Check sheet for the drawn part. Datum: minimum x, y, z corner. Units: mm. A direction names the side the tool comes from. Round coordinates to 2 decimals unless told otherwise and drop trailing zeros. Order: outer loops, then holes, each group sorted by start corner. A loop starts at its lowest first (then second) coordinate and runs counter-clockwise, first axis right, second up. Notation, with made-up numbers: M 1,-1.75 L 43,-1.75 A11 cw 43,11.25 Z; hole C 84.25,34.25 d10. An arc over 180 degrees is marked long. Answer as a JSON object with one key per item and string values. Group by question number.
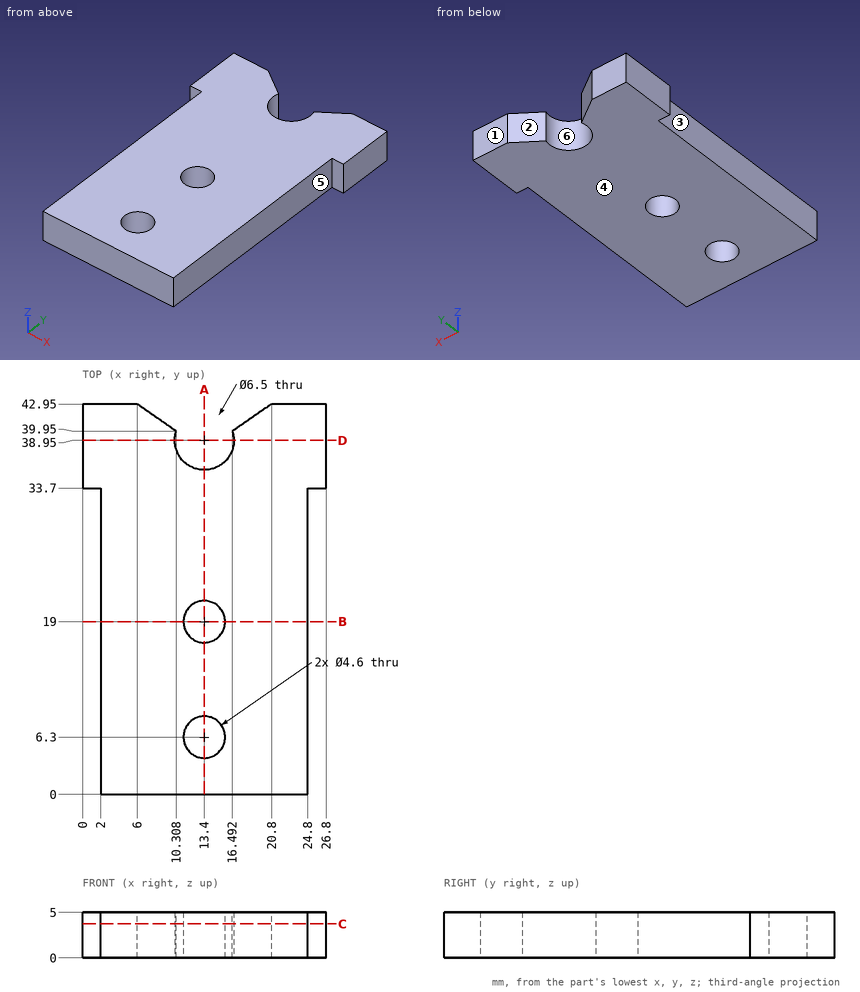
1) Go/stop test with flat-tipped pins: P1, Ø1, axis at x = 18.5, z = 3.5, coming from the +Y side; P2, Ø1.6, axis at x = 26, z = 2, coming from the -Y side; P3, Ø1.5, axis at y = 11, z = 3, coming from the -X side. Record where each tip stops, or that it passes through.
2) Set-up check for the marked faces 1, 2 and 3: record each of +Z, -Z, +X, -X, +Y, -Y from which the full face is reachable in a straight line by a thin tool's end or side.
3) Sectioned sample at A-A (x = 13.4). Record the boundary of the cut face in (y, z).
4) Release check for a two-part mould opening along X. For the marked faces 4, 5 and 6 record: +X half, -X half, draft (parallel to the pull), parting line (faces both ways), or undercut.
5) Thickness scan on line 1 along Y through (x, z) = (13.4, 2.9); line 2 along X through (y, z) = (6.5, 3.3); line 3 along Y through (x, z) = (15.5, 1.1) (1 decimal). Record the ranges inside material, lowest first. Write a range as [from, to].
6) Sectioned sample at D-D (y = 38.95). Record the boundary of the cut face in (x, z), then the cut area to 4 significant figures.
7) Sectioned sample at C-C (z = 3.75). Record the boundary of the cut face in (x, y).
8) Sectioned sample at B-B (y = 19). Record the boundary of the cut face in (x, z), then the cut area to 3 significant figures.
Final values:
{
 "1": {"P1": "stops at y = 41.7", "P2": "stops at y = 33.7", "P3": "stops at x = 2"},
 "2": {"face 1": "+Z, -Z, +X, -X, +Y", "face 2": "+Z, -Z, +Y", "face 3": "+Z, -Z, -X, -Y"},
 "3": {"outline": "M 0,0 L 4,0 L 4,5 L 0,5 Z; M 8.6,0 L 16.7,0 L 16.7,5 L 8.6,5 Z; M 21.3,0 L 35.7,0 L 35.7,5 L 21.3,5 Z"},
 "4": {"face 4": "draft", "face 5": "+X half", "face 6": "undercut"},
 "5": {"line 1": "y = [0, 4], [8.6, 16.7], [21.3, 35.7]", "line 2": "x = [2, 11.11], [15.69, 24.8]", "line 3": "y = [0, 5.4], [7.2, 18.1], [19.9, 36.5]"},
 "6": {"outline": "M 0,0 L 10.15,0 L 10.15,5 L 0,5 Z; M 16.65,0 L 26.8,0 L 26.8,5 L 16.65,5 Z", "area": "101.5 mm^2"},
 "7": {"outline": "M 0,33.7 L 2,33.7 L 2,0 L 24.8,0 L 24.8,33.7 L 26.8,33.7 L 26.8,42.95 L 20.8,42.95 L 16.49,39.95 A3.25 cw long 10.31,39.95 L 6,42.95 L 0,42.95 Z; hole C 13.4,6.3 d4.6; hole C 13.4,19 d4.6"},
 "8": {"outline": "M 2,0 L 11.1,0 L 11.1,5 L 2,5 Z; M 15.7,0 L 24.8,0 L 24.8,5 L 15.7,5 Z", "area": "91.0 mm^2"}
}
